```python
from build123d import *

# Parameters (mm, degrees)
F0_R     = 100
F0_R_2   = 27
F1_DEPTH = 3.5
F2_R     = 45
F2_R_2   = 27
F3_DEPTH = 61
F4_R     = 100
F4_R_2   = 27
F5_DEPTH = 3.5


with BuildPart() as f1:
    # F0 (on Front) → F1 (new body)
    with BuildSketch(Plane.XZ):
        Circle(F0_R)
        Circle(F0_R_2, mode=Mode.SUBTRACT)
    extrude(amount=F1_DEPTH)

    # F2 (on face) → F3 (join)
    with BuildSketch(Plane(origin=(0, 0, 0), x_dir=(-1, 0, 0), z_dir=(0, 1, 0))):
        Circle(F2_R)
        Circle(F2_R_2, mode=Mode.SUBTRACT)
    extrude(amount=F3_DEPTH)

    # F4 (on face) → F5 (join)
    with BuildSketch(Plane(origin=(0, 61, 0), x_dir=(-1, 0, 0), z_dir=(0, 1, 0))):
        Circle(F4_R)
        Circle(F4_R_2, mode=Mode.SUBTRACT)
    extrude(amount=F5_DEPTH)


solid = f1.part
```
Input: part model. Units: mm. Frame: model coordinates. A direction names the side the tool comes from. Round coordinates to 2 decimals unless told otherwise and drop trailing zeros. Write each loop counter-clockwise with the first axis right and the second up, starting at its lowest first coordinate (ties: lowest second). Pieces come first, ordered by that corner, then holes. Notation, with made-up numbers: (4, 42) - (47, 42) arc R19 cw to (47, 61) - close; hole circle Ø1 at (10.5, -26). An arc over 180 degrees is marked (long way). Write item = value, one per line.
(1) Section query A-A on x = 0. Output: boundary loops of the cut face in (y, z), then the cut area to 3 significant figures.
Geometry check:
outline = (-3.5, -100) - (0, -100) - (0, -45) - (61, -45) - (61, -100) - (64.5, -100) - (64.5, -27) - (-3.5, -27) - close; (-3.5, 27) - (64.5, 27) - (64.5, 100) - (61, 100) - (61, 45) - (0, 45) - (0, 100) - (-3.5, 100) - close
area = 3,220 mm^2
(2) Access query for faces 5 (the flat face through (-21, 61, -43)), 6 (the cylindrical face through (95.38, -1.73, 30.04)). Directions: +Z, -Z, +X, -X, +Y, -Y. A direction counts if a zero-diameter tool reaches every point of the face in a straight line with its end or side. Return the directions, or none.
Geometry check:
face_5 = none
face_6 = +Y, -Y
(3) Material intervals for probe 1 along Z at (x, y) = (0, -1.3); probe 2 along Y at (x, z) = (64.5, 11); probe 3 along X at (y, z) = (22.5, 7.5), sorted ascending.
Geometry check:
probe_1 = -100 to -27, 27 to 100
probe_2 = -3.5 to 0, 61 to 64.5
probe_3 = -44.37 to -25.94, 25.94 to 44.37
(4) Contact query for flat-ended pins moving along their axis: pin 1 Ø10 at (x, y) = (-23.5, 42.5) entering from -Z; pin 2 Ø3 at (y, z) = (23, 41.5) entering from +X. Output: stop coordinate, or through.
Geometry check:
pin_1 = -41.02
pin_2 = 20.62
(5) Pull-direction query (Y, two-part tool) for faces 1 (the flat face through (-21, 64.5, -21)), 2 (the flat face through (21, -3.5, -21)), 3 (the cylindrical face through (-95.38, 62.73, 30.04)), 4 (the flat face through (21, 0, -43)); classes: +Y half, -Y half, draft (parallel to the pull), parting line (faces both ways), or undercut.
Geometry check:
face_1 = +Y half
face_2 = -Y half
face_3 = draft
face_4 = undercut
(6) Section query B-B on z = -87. Output: boundary loops of the cut face in (x, y), then the cut area to 3 significant figures.
Geometry check:
outline = (-49.31, -3.5) - (49.31, -3.5) - (49.31, 0) - (-49.31, 0) - close; (-49.31, 61) - (49.31, 61) - (49.31, 64.5) - (-49.31, 64.5) - close
area = 690 mm^2
(7) Section query C-C on y = 51. Output: boundary loops of the cut face in (x, z).
Geometry check:
outline = circle Ø90 at (0, 0); hole circle Ø54 at (0, 0)
(8) Section query D-D on x = -24. Output: boundary loops of the cut face in (y, z).
Geometry check:
outline = (-3.5, -97.08) - (0, -97.08) - (0, -38.07) - (61, -38.07) - (61, -97.08) - (64.5, -97.08) - (64.5, -12.37) - (-3.5, -12.37) - close; (-3.5, 12.37) - (64.5, 12.37) - (64.5, 97.08) - (61, 97.08) - (61, 38.07) - (0, 38.07) - (0, 97.08) - (-3.5, 97.08) - close
